Part print with two shaded views. Sizes in mm from the minimum x, y, z corner. A direction names the side the tool comes from. Coordinates: 2 decimals unless noted, no trailing zeros. Write each loop counter-clockwise with the first axis right and the second up, starting at its lowest first coordinate (ties: lowest second). Pieces come first, ordered by that corner, then holes. Notation, with made-up numbers: (15, 35.5) - (23, 35.5) arc R11 ccw to (23, 50.5) - close; hole circle Ø1 at (-22, 32.5). An arc over 180 degrees is marked (long way). One line per question, with ' | ' between items. Start each with the question number.
1. Band-saw the part on A-A, the plane y = 8.25. Write the cut outline in (x, z) (1 decimal), then the cut area to 3 significant figures.
2. Flat gauge pins, fed straight in: P1, Ø1, axis at y = 3, z = 3, coming from the +X side; P2, Ø1.5, axis at x = 7.5, y = 4, coming from the -Z side; P3, Ø1, axis at y = 15.5, z = 1, coming from the -X side (1 decimal). Where does each tip first touch, or does it go through?
3. Which spindle directions (+Z, -Z, +X, -X, +Y, -Y) get a long thin tool onto all of the face, cutting with end or side? Do the marked faces 1, 2, 3 and 4. Say none if no direction does.
4. Band-saw the part on C-C, the plane x = 10.25. Write the cut outline in (y, z).
5. Probe line 1 (Y direction, x = 6, z = 1.9); line 2 (X direction, y = 14, z = 2.1) (1 decimal); line 3 (X direction, y = 2, z = 1.45) (1 decimal). List the from-to ranges inside material, lowest first.
6. Band-saw the part on D-D, the plane y = 2.5. Write the cut outline in (x, z) (1 decimal).
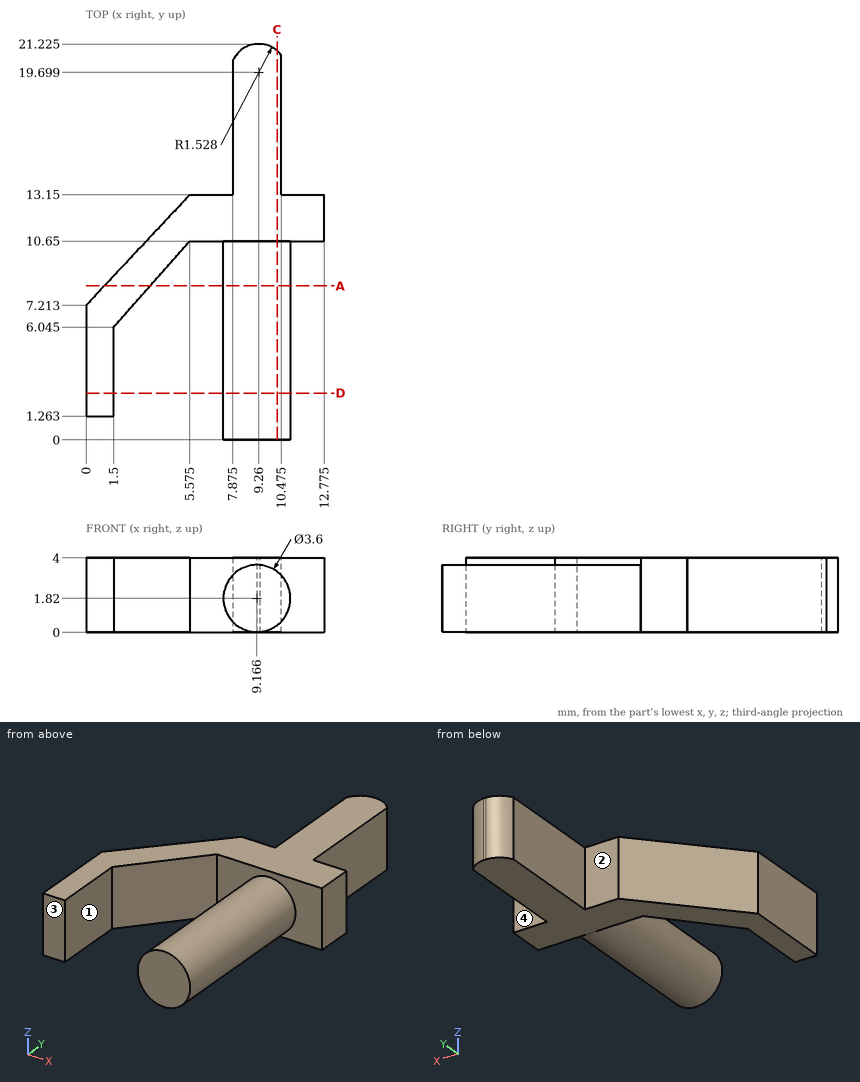
Filled in:
1) outline: (1, 0) - (3.5, 0) - (3.5, 4) - (1, 4) - close; circle Ø3.6 at (9.2, 1.8) | area: 20.1 mm²
2) P1: stops at x = 10.83 | P2: stops at z = 0.27 | P3: stops at x = 7.9
3) face 1: +Z, -Z, -Y | face 2: +Z, -Z, -X, +Y | face 3: +Z, -Z, -X, -Y | face 4: +Z, -Z, +X, +Y
4) outline: (0, 0.38) - (10.65, 0.38) - (10.65, 0) - (20.86, 0) - (20.86, 4) - (10.65, 4) - (10.65, 3.26) - (0, 3.26) - close
5) line 1: y = 10.65 to 13.15 | line 2: x = 7.9 to 10.5 | line 3: x = 0 to 1.5, 7.4 to 10.9
6) outline: (0, 0) - (1.5, 0) - (1.5, 4) - (0, 4) - close; circle Ø3.6 at (9.2, 1.8)
